```python
from build123d import *

# Parameters (mm, degrees)
RESSALTO_EXTRUS_O1_DEPTH = 0.3


with BuildPart() as part:
    # Esboço1 → Ressalto-extrusão1 (new body, symmetric)
    with BuildSketch(Plane.XY):
        with BuildLine():
            Line((18.8, 0.2), (18.8, 0))
            Line((18.8, 0), (18, 0))
            ThreePointArc((18, 0), (17.90513167, 0.015395011), (17.82, 0.06))
            Line((17.82, 0.06), (16.946446609, 0.970710678))
            ThreePointArc((16.946446609, 0.970710678), (16.914021314, 0.992429091), (16.875735931, 1))
            Line((16.875735931, 1), (12.407488688, 0.99))
            Line((12.407488688, 0.99), (10.557971552, 1.813458083))
            ThreePointArc((10.557971552, 1.813458083), (10.373577052, 1.832838725), (10.213007112, 1.740133627))
            Line((10.213007112, 1.740133627), (9.099531826, 0.503494039))
            Line((9.099531826, 0.503494039), (8.95090286, 0.637320161))
            Line((8.95090286, 0.637320161), (10.064378147, 1.873959748))
            ThreePointArc((10.064378147, 1.873959748), (10.331994714, 2.028468246), (10.639318881, 1.996167174))
            Line((10.639318881, 1.996167174), (12.45, 1.19))
            Line((12.45, 1.19), (16.875735931, 1.2))
            ThreePointArc((16.875735931, 1.2), (16.990592571, 1.177288457), (17.087867966, 1.112132034))
            Line((17.087867966, 1.112132034), (17.937254364, 0.258898547))
            ThreePointArc((17.937254364, 0.258898547), (18.002249513, 0.215310679), (18.078994902, 0.2))
            Line((18.078994902, 0.2), (18.8, 0.2))
        make_face()
    extrude(amount=RESSALTO_EXTRUS_O1_DEPTH, both=True)


solid = part.part
```
Part model, mm, in its own coordinate system. Round coordinates to 2 decimals unless told otherwise and drop trailing zeros. Order: outer loops, then holes, each group sorted by start corner. A loop starts at its lowest first (then second) coordinate and runs counter-clockwise, first axis right, second up. Notation, with made-up numbers: M -38.5,-26.5 L -6.5,-26.5 A26 cw -6.5,11.5 Z; hole C 45.5,71.5 d5. An arc over 180 degrees is marked long. Put each result on its own line as item: value. Start each with the question number.
1. Slice it at C-C on x = 12. List the corners of the cut face in (y, z).
2. Slice it at B-B on y = 0.35. List the corners of the cut face in (x, z), then the cut area to 3 significant figures.
3. Drill centre lines: probe 1 along Y at (x, z) = (13, -0.1); probe 2 along X at (y, z) = (0.7, 0.05); probe 3 along X at (y, z) = (0.8, -0.2). Where is each one in solid material? Low to high. Write a range as [from, to].
4. Slice it at A-A on z = -0.2. List the corners of the cut face in (x, y), then the cut area to 3 significant figures.
5. Two-plate mould, pull along X, no slides. Class faces 1 (the face through (9.5, 1.25, 0)), 2 (the face through (17.5, 0.7, 0)), 3 (the face through (11.496, 1.396, 0.004)): +X half, -X half, draft (parallel to the pull), parting line (faces both ways), or undercut.
Findings:
1. outline: M 1.17,-0.3 L 1.39,-0.3 L 1.39,0.3 L 1.17,0.3 Z
2. outline: M 17.54,-0.3 L 17.85,-0.3 L 17.85,0.3 L 17.54,0.3 Z
2. area: 0.183 mm2
3. probe 1: [0.99, 1.19]
3. probe 2: [9.01, 9.28], [17.21, 17.5]
3. probe 3: [9.1, 9.37], [17.11, 17.4]
4. outline: M 8.95,0.64 L 9.1,0.5 L 10.21,1.74 A0.3 cw 10.56,1.81 L 12.41,0.99 L 16.88,1 A0.1 cw 16.95,0.97 L 17.82,0.06 A0.3 ccw 18,0 L 18.8,0 L 18.8,0.2 L 18.08,0.2 A0.2 cw 17.94,0.26 L 17.09,1.11 A0.3 ccw 16.88,1.2 L 12.45,1.19 L 10.64,2 A0.5 ccw 10.06,1.87 Z
4. area: 2.21 mm2
5. face 1: -X half
5. face 2: +X half
5. face 3: undercut
